Drawing for the job (mm, zero at the part's lowest x, y, z). A direction names the side the tool comes from. Coordinates: 2 decimals unless noted, no trailing zeros. Order: outer loops, then holes, each group sorted by start corner. A loop starts at its lowest first (then second) coordinate and runs counter-clockwise, first axis right, second up. Notation, with made-up numbers: (-38, 83.25) - (0, 83.25) arc R31 cw to (0, 112.25) - close; hole circle Ø2 at (26, 2). An arc over 180 degrees is marked (long way). Put each result on its own line as item: value. Start each with the question number.
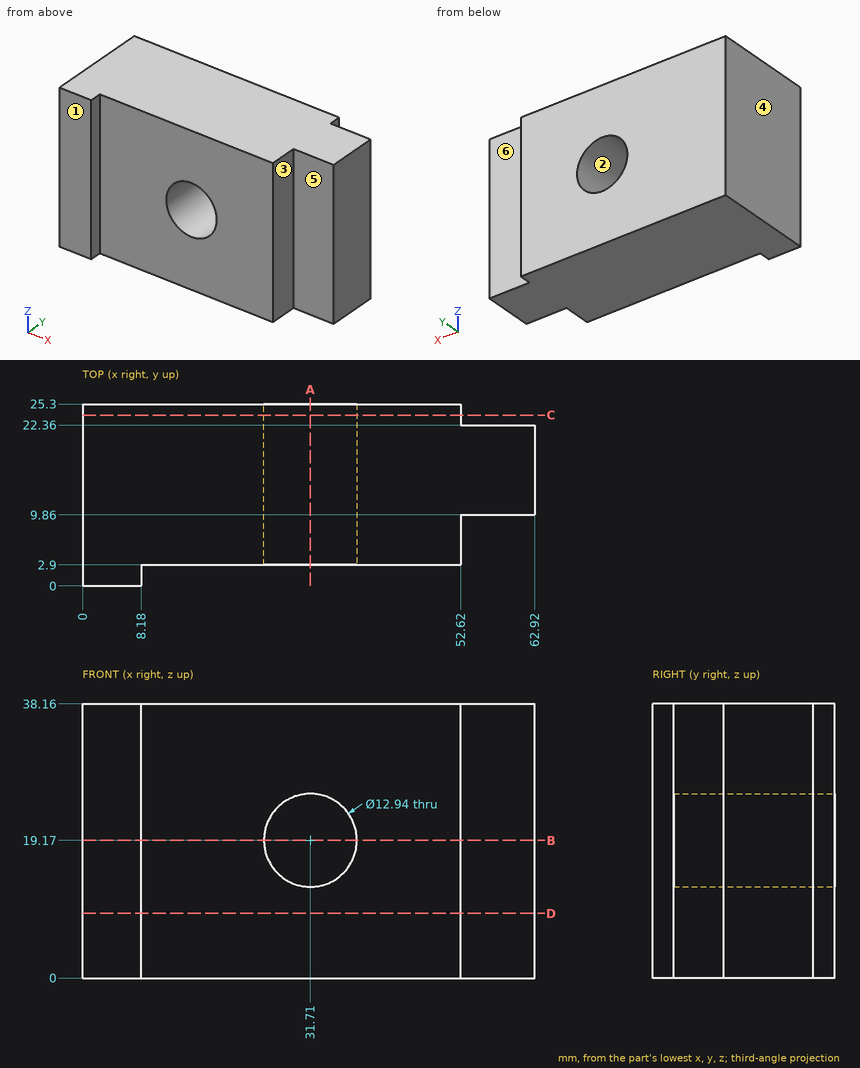
Item 1: 3-axis set-ups, long thin cutter, end or side, ignore diameter. For the marked faces 4, 5 and 6: which of +Z, -Z, +X, -X, +Y, -Y reach the whole face in a straight line?
Item 2: Slice it at C-C, the plane y = 23.75. Give the cut face in (x, z), plus the area to 3 significant figures.
Item 3: Slice it at D-D, the plane z = 9. Give the cut face in (x, y).
Item 4: Pull direction X, two halves, no side cores. Call the marked faces 1, 2 and 3: pulls with the +X half, pulls with the -X half, needs draft (parallel to the pull), parting line crosses it, or undercut.
Item 5: Flat gauge pins, fed straight in: pin 1 Ø19 at (x, z) = (35, 19.5) entering from -Y; pin 2 Ø12 at (x, y) = (39, 3.5) entering from -Z; pin 3 Ø5 at (x, z) = (59.5, 23.5) entering from -Y; pin 4 Ø7.5 at (y, z) = (5.5, 9.5) entering from +X. Where does each tip first touch, or does it go through?
Item 6: Wall check: line 1 along Z through (x, y) = (31.71, 12.25); line 2 along Y through (x, z) = (14.5, 11); line 3 along X through (y, z) = (8.25, 8). Give the ranges that are in metal, low to high.
Item 7: Slice it at A-A, the plane x = 31.71. Give the cut face in (y, z).
Item 8: Slice it at B-B, the plane z = 19.17. Give the cut face in (x, y), plus the area to 3 significant figures.
Here are the results:
1. face 4: +Z, -Z, -X, +Y, -Y
1. face 5: +Z, -Z, +X, -Y
1. face 6: +Z, -Z, +X, +Y
2. outline: (0, 0) - (52.62, 0) - (52.62, 38.16) - (0, 38.16) - close; hole circle Ø12.94 at (31.71, 19.17)
2. area: 1,880 mm^2
3. outline: (0, 0) - (8.18, 0) - (8.18, 2.9) - (52.62, 2.9) - (52.62, 9.86) - (62.92, 9.86) - (62.92, 22.36) - (52.62, 22.36) - (52.62, 25.3) - (0, 25.3) - close
4. face 1: needs draft
4. face 2: undercut
4. face 3: pulls with the +X half
5. pin 1: stops at y = 2.9
5. pin 2: stops at z = 0
5. pin 3: stops at y = 9.86
5. pin 4: stops at x = 52.62
6. line 1: z = 0 to 12.7, 25.64 to 38.16
6. line 2: y = 2.9 to 25.3
6. line 3: x = 0 to 52.62
7. outline: (2.9, 0) - (25.3, 0) - (25.3, 12.7) - (2.9, 12.7) - close; (2.9, 25.64) - (25.3, 25.64) - (25.3, 38.16) - (2.9, 38.16) - close
8. outline: (0, 0) - (8.18, 0) - (8.18, 2.9) - (25.24, 2.9) - (25.24, 25.3) - (0, 25.3) - close; (38.18, 2.9) - (52.62, 2.9) - (52.62, 9.86) - (62.92, 9.86) - (62.92, 22.36) - (52.62, 22.36) - (52.62, 25.3) - (38.18, 25.3) - close
8. area: 1,040 mm^2
